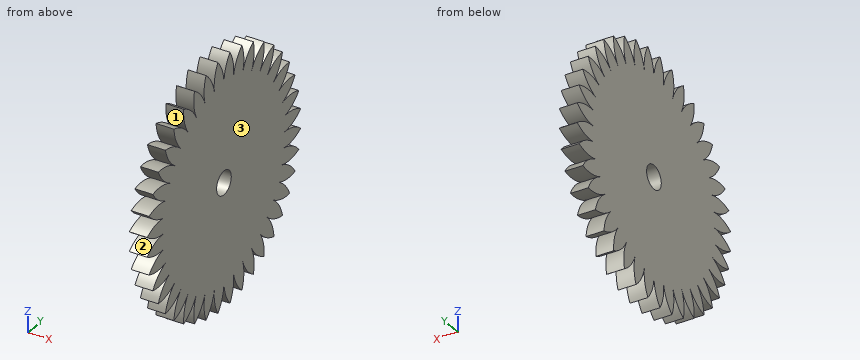
```python
from build123d import *

# Parameters (mm, degrees)
BOSS_EXTRUDE1_DEPTH = 3
CIRPATTERN1_COUNT   = 40
SKETCH2_R           = 2
CUT_EXTRUDE2_DEPTH  = 4


with BuildPart() as part:
    # Sketch1 → Boss-Extrude1 (new body)
    with BuildSketch(Plane(origin=(0, 0, 0), x_dir=(0, 0, -1), z_dir=(1, 0, 0))):
        with BuildLine():
            Line((0, 16.5), (0, 0))
            Line((0, 0), (2.581168673, 16.29685762))
            ThreePointArc((2.581168673, 16.29685762), (2.531264023, 18.699958072), (1.64764101, 20.935264008))
            ThreePointArc((1.64764101, 20.935264008), (0.425217975, 18.865707491), (0, 16.5))
        make_face()
    boss_extrude1 = extrude(amount=BOSS_EXTRUDE1_DEPTH)

    # CirPattern1: Boss-Extrude1 ×40 about axis
    cirpattern1_axis = Axis((0, 0, 0), (1, 0, 0))
    for i in range(1, CIRPATTERN1_COUNT):
        add(boss_extrude1.rotate(cirpattern1_axis, i * 360 / CIRPATTERN1_COUNT))

    # Sketch2 → Cut-Extrude2 (cut, through all)
    with BuildSketch(Plane(origin=(0, 0, 0), x_dir=(0, 0, -1), z_dir=(1, 0, 0))):
        Circle(SKETCH2_R)
    extrude(amount=CUT_EXTRUDE2_DEPTH, mode=Mode.SUBTRACT)


solid = part.part
```
Verification items for the finished model (mm, model axes). Face numbers are marked on the shaded views. Give positions to 0.01 mm unless a question says otherwise; leave off trailing zeros. Order: outer loops, then holes, each group sorted by start corner. A loop starts at its lowest first (then second) coordinate and runs counter-clockwise, first axis right, second up. Notation, with made-up numbers: (4.25, 54) -> (52.25, 54) arc R13 cw to (52.25, 69) -> close; hole circle Ø5 at (-30.5, 24.25). An arc over 180 degrees is marked (long way). One line per item, written item: value.
(1) Sectioned sample at A-A on z = 12.5. Record the cut outline in (x, y).
Final values:
outline: (0, -15.59) -> (3, -15.59) -> (3, -12.68) -> (0, -12.68) -> close; (0, -12.38) -> (3, -12.38) -> (3, 12.38) -> (0, 12.38) -> close; (0, 12.68) -> (3, 12.68) -> (3, 15.59) -> (0, 15.59) -> close
(2) Sectioned sample at C-C on z = -4. Record the cut outline in (x, y).
Final values:
outline: (0, -19.5) -> (3, -19.5) -> (3, 19.5) -> (0, 19.5) -> close
(3) Sectioned sample at B-B on y = -17. Count the separate pieces of the cut face and the enclosed holes in it, then the cut area to 3 significant figures.
Final values:
separate pieces: 8
enclosed holes: 0
area: 56.3 mm^2
(4) Draft check along Z on the marked faces 1, 2 and 3. Enter one of: pulls with the +Z half, pulls with the -Z half, needs draft (parallel to the pull), parting line crosses it, or undercut.
Final values:
face 1: undercut
face 2: undercut
face 3: needs draft
(5) Gauge pin test, flat ends, axial feed: pin 1 (2.5 mm diameter, centred on y = 0, z = 0, fed in from -X); pin 2 (1.5 mm diameter, centred on x = 2, y = 16.5, fed in from +Z); pin 3 (1 mm diameter, centred on x = 1, y = -16, fed in from -Z). Record the tip position at first contact, or that the pin passes through.
Final values:
pin 1: through
pin 2: z = 13.64
pin 3: z = -13.64
(6) Scan lines: line 1 along Z through (x, y) = (1, -19); line 2 along Z through (x, y) = (0.1, 13); line 3 along Z through (x, y) = (1.3, 19.5). Record each from-to range of solid material in increasing order. Write a range as [from, to].
Final values:
line 1: [-8.12, -7.45], [-5.32, -3.64], [-2.46, -0.48], [0.48, 2.46], [3.64, 5.32], [7.45, 8.12]
line 2: [-15.78, -13.56], [-12.7, 12.7], [13.56, 15.78]
line 3: [-5.21, -4], [-2.32, -0.7], [0.7, 2.32], [4, 5.21]
